Read the model definition and answer for the solid it produces. Units are mm, in the model's axes. Face numbers are marked on the shaded views. A direction names the side the tool comes from. Coordinates: 2 decimals unless noted, no trailing zeros. Write each loop counter-clockwise with the first axis right and the second up, starting at its lowest first coordinate (ties: lowest second). Pieces come first, ordered by that corner, then holes. Notation, with made-up numbers: (-39, 10.5) -> (-1, 10.5) arc R28 ccw to (-1, 41.5) -> close; hole circle Ø1 at (-19, 31.5). An arc over 180 degrees is marked (long way). One line per item, written item: value. Start each with the question number.
1. For the marked faces 1, 2 and 3, determine the directions among +Z, -Z, +X, -X, +Y, -Y from which every point of the face is accessible in a straight line to the end or side of a thin tool.
2. Given P1, Ø1.8, axis at x = -0.5, y = -144.5, coming from the +Z side, flat-ended and moving along its own axis, determine where the tip first touches the part or whether it passes through.
3. Find section B-B, the plane x = -1.75. Write down the section's boundary in (y, z).
4. Consider line 1 along Y through (x, z) = (3.5, -2). Determine where the line is inside the solid, lowest interval first.
5. Find section A-A, the plane z = -0.75. Write down the section's boundary in (x, y), and give its area (3 significant figures).
Solid Edge part; units mm, degrees
sketch "Sketch1" plane through (0, 0, 0) normal (0, -1, 0) x (1, 0, 0)
  line L0 (-4, 4) -> (4, 4)
  line L1 (4, 4) -> (4, -4)
  line L2 (4, -4) -> (-4, -4)
  line L3 (-4, -4) -> (-4, 4)
  dimension "D1" = 4
  dimension "D2" = 4
extrude "Protrusion1" add sketch "Sketch1" along normal blind 150
sketch "Sketch2" plane through (0, -150, 0) normal (0, -1, 0) x (1, 0, 0)
  line L0 (-3, 3) -> (3, 3)
  line L1 (3, 3) -> (3, -3)
  line L2 (3, -3) -> (-3, -3)
  line L3 (-3, -3) -> (-3, 3)
  line L4 (-4, -4) -> (4, -4)
  line L5 (4, -4) -> (4, 4)
  line L6 (4, 4) -> (-4, 4)
  line L7 (-4, 4) -> (-4, -4)
  dimension "D1" = 3
extrude "Extrusionsausschnitt_1" cut sketch "Sketch2" against normal blind 10
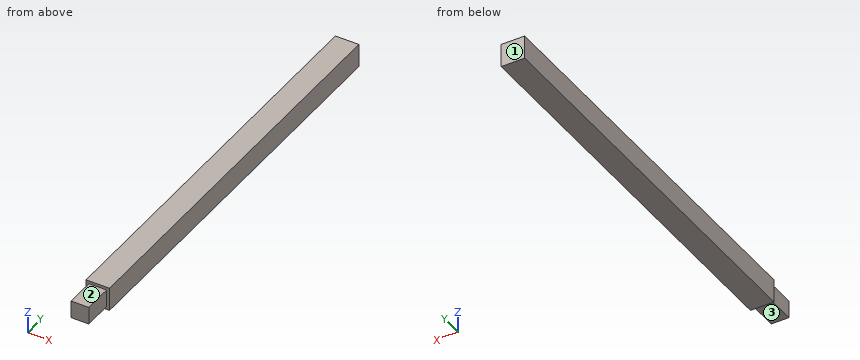
Answer block:
1. face 1: +Z, -Z, +X, -X, +Y
1. face 2: +Z, +X, -X, -Y
1. face 3: -Z, +X, -X, -Y
2. P1: stops at z = 3
3. outline: (-150, -3) -> (-140, -3) -> (-140, -4) -> (0, -4) -> (0, 4) -> (-140, 4) -> (-140, 3) -> (-150, 3) -> close
4. line 1: y = -140 to 0
5. outline: (-4, -140) -> (-3, -140) -> (-3, -150) -> (3, -150) -> (3, -140) -> (4, -140) -> (4, 0) -> (-4, 0) -> close
5. area: 1,180 mm2
